```python
from build123d import *

# Parameters (mm, degrees)
SKETCH1_W           = 35
SKETCH1_H           = 15
BOSS_EXTRUDE1_DEPTH = 23.49
SKETCH2_W           = 22.56001237
SKETCH2_H           = 32.900224363
SKETCH2_W_2         = 23.005303498
CUT_EXTRUDE1_DEPTH  = 23.49
SKETCH3_W           = 17
SKETCH3_H           = 15.731554352
CUT_EXTRUDE2_DEPTH  = 23.49
SKETCH5_W           = 8.6
SKETCH5_H           = 9
CUT_EXTRUDE4_DEPTH  = 12.5
SKETCH8_W           = 12.842835289
SKETCH8_H           = 9
CUT_EXTRUDE5_DEPTH  = 10.5
SKETCH4_R           = 2.5
CUT_EXTRUDE6_DEPTH  = 5.107289171
SKETCH9_R           = 1.5
CUT_EXTRUDE7_DEPTH  = 16


with BuildPart() as part:
    # Sketch1 → Boss-Extrude1 (new body)
    with BuildSketch(Plane(origin=(0, 0, 0), x_dir=(1, 0, 0), z_dir=(0, 1, 0))):
        with Locations((17.5, 7.5)):
            Rectangle(SKETCH1_W, SKETCH1_H)
    extrude(amount=BOSS_EXTRUDE1_DEPTH)

    # Sketch2 → Cut-Extrude1 (cut)
    with BuildSketch(Plane.XY):
        with Locations((37.280006185, 20.557401353)):
            Rectangle(SKETCH2_W, SKETCH2_H)
        with Locations((-2.502651749, 20.557401353)):
            Rectangle(SKETCH2_W_2, SKETCH2_H)
    extrude(amount=-CUT_EXTRUDE1_DEPTH, mode=Mode.SUBTRACT)

    # Sketch3 → Cut-Extrude2 (cut)
    with BuildSketch(Plane.XY):
        with Locations((17.5, 23.355777176)):
            Rectangle(SKETCH3_W, SKETCH3_H)
    extrude(amount=-CUT_EXTRUDE2_DEPTH, mode=Mode.SUBTRACT)

    # Sketch5 → Cut-Extrude4 (cut)
    with BuildSketch(Plane(origin=(0, 15.49, 0), x_dir=(1, 0, 0), z_dir=(0, 1, 0))):
        with Locations((17.5, 7.5)):
            Rectangle(SKETCH5_W, SKETCH5_H)
    extrude(amount=-CUT_EXTRUDE4_DEPTH, mode=Mode.SUBTRACT)

    # Sketch8 → Cut-Extrude5 (cut)
    with BuildSketch(Plane(origin=(0, 2.99, 0), x_dir=(1, 0, 0), z_dir=(0, 1, 0))):
        with Locations((17.535477445, 7.5)):
            Rectangle(SKETCH8_W, SKETCH8_H)
    extrude(amount=CUT_EXTRUDE5_DEPTH, mode=Mode.SUBTRACT)

    # Sketch4 → Cut-Extrude6 (cut, through all)
    with BuildSketch(Plane(origin=(0, 4.107289171, 0), x_dir=(1, 0, 0), z_dir=(0, 1, 0))):
        with Locations((4.5, 7.5)):
            Circle(SKETCH4_R)
        with Locations((30.5, 7.5)):
            Circle(SKETCH4_R)
    extrude(amount=-CUT_EXTRUDE6_DEPTH, mode=Mode.SUBTRACT)

    # Sketch9 → Cut-Extrude7 (cut, through all)
    with BuildSketch(Plane.XY):
        with Locations((17.5, 7.780477446)):
            Circle(SKETCH9_R)
    extrude(amount=-CUT_EXTRUDE7_DEPTH, mode=Mode.SUBTRACT)


solid = part.part
```
The listing builds one solid part. Answer for the finished solid, in the listing's coordinates (mm). A direction names the side the tool comes from. Give positions to 0.01 mm unless a question says otherwise; leave off trailing zeros. Write each loop counter-clockwise with the first axis right and the second up, starting at its lowest first coordinate (ties: lowest second). Pieces come first, ordered by that corner, then holes. Notation, with made-up numbers: (19.25, 42.25) -> (27.25, 42.25) arc R22 ccw to (27.25, 62.25) -> close; hole circle Ø9 at (84.5, 36.5). An arc over 180 degrees is marked (long way). Use one line per item in the form item = value.
1) Section C-C on y = 13 is taken. Write down the section's boundary in (x, z), plus the area to 3 significant figures.
Result:
outline = (9, -15) -> (26, -15) -> (26, 0) -> (9, 0) -> close; hole (11.11, -12) -> (23.96, -12) -> (23.96, -3) -> (11.11, -3) -> close
area = 139 mm²
2) Section B-B on x = 17.5 is taken. Write down the section's boundary in (y, z), plus the area to 3 significant figures.
Result:
outline = (0, -15) -> (6.28, -15) -> (6.28, -12) -> (2.99, -12) -> (2.99, -3) -> (6.28, -3) -> (6.28, 0) -> (0, 0) -> close; (9.28, -15) -> (15.49, -15) -> (15.49, -12) -> (9.28, -12) -> close; (9.28, -3) -> (15.49, -3) -> (15.49, 0) -> (9.28, 0) -> close
area = 102 mm²
3) Section A-A on z = -7.5 is taken. Write down the section's boundary in (x, y), plus the area to 3 significant figures.
Result:
outline = (0, 0) -> (2, 0) -> (2, 4.11) -> (0, 4.11) -> close; (7, 0) -> (28, 0) -> (28, 4.11) -> (26, 4.11) -> (26, 15.49) -> (21.8, 15.49) -> (21.8, 13.49) -> (23.96, 13.49) -> (23.96, 2.99) -> (11.11, 2.99) -> (11.11, 13.49) -> (13.2, 13.49) -> (13.2, 15.49) -> (9, 15.49) -> (9, 4.11) -> (7, 4.11) -> close; (33, 0) -> (35, 0) -> (35, 4.11) -> (33, 4.11) -> close
area = 144 mm²
4) For a pull along Z with two mould halves and no side action, classify faces 1 (the flat face through (17, 6, -15)), 2 (the cylindrical face through (5.65, 2.08, -5.28)), 3 (the flat face through (17, 6, 0)), 4 (the flat face through (17, 0, -8)) as +Z half, -Z half, draft (parallel to the pull), parting line (faces both ways), or undercut.
Result:
face_1 = -Z half
face_2 = undercut
face_3 = +Z half
face_4 = draft
5) Section D-D on x = 30.5 is taken. Write down the section's boundary in (y, z).
Result:
outline = (0, -15) -> (4.11, -15) -> (4.11, -10) -> (0, -10) -> close; (0, -5) -> (4.11, -5) -> (4.11, 0) -> (0, 0) -> close
6) Straight lines are drawn through the part: probe 1 along X at (y, z) = (2.1, -7.5); probe 2 along Y at (x, z) = (22, -8.25); probe 3 along X at (y, z) = (7, -8.75). For each, find the intervals that lie inside material, in ascending order.
Result:
probe_1 = 0 to 2, 7 to 28, 33 to 35
probe_2 = 0 to 2.99, 13.49 to 15.49
probe_3 = 9 to 11.11, 23.96 to 26
7) A tool of negligible diameter and unlimited length cuts with its end or side. For faces 5 (the flat face through (13.2, 15, -7)), 6 (the flat face through (2, 4.107, -6)), 7 (the flat face through (23, 13.49, -8)), 8 (the flat face through (26, 10, -7)), from which of +Z, -Z, +X, -X, +Y, -Y can it reach the whole face along a straight path? Write none if from no direction.
Result:
face_5 = +Y
face_6 = +Z, -Z, -X, +Y
face_7 = none
face_8 = +Z, -Z, +X, +Y
8) Each of these flat-tipped pins is pushed along its axis until it touches: P1, Ø4.5, axis at y = 8.5, z = -6, coming from the +X side; P2, Ø1, axis at y = 15, z = -7.5, coming from the -X side; P3, Ø2.5, axis at x = 17.5, z = -5.5, coming from the +Y side. Where does it stop, or does it pass through?
Result:
P1 = 26
P2 = 9
P3 = 2.99
